Source: CAD feature listing. Evaluate the final solid. Frame: model axes, mm. Give positions to 0.01 mm unless a question says otherwise; leave off trailing zeros. Order: outer loops, then holes, each group sorted by start corner. A loop starts at its lowest first (then second) coordinate and runs counter-clockwise, first axis right, second up. Notation, with made-up numbers: M 17,-9 L 32,-9 A26 cw 32,11 Z; hole C 11,64 d11. An arc over 180 degrees is marked long. One line per question, with ' | ' between items. Start each with the question number.
from build123d import *

# Parameters (mm, degrees)
SKETCH1_R                                       = 335
SKETCH1_R_2                                     = 295
BOSS_EXTRUDE1_DEPTH                             = 8.5
CBORE_FOR_M4_SHCS1_D                            = 4.5
CBORE_FOR_M4_SHCS1_CBORE_D                      = 8
CBORE_FOR_M4_SHCS1_CBORE_DEPTH                  = 4
CSK_FOR_M4_FLAT_HEAD_MACHINE_SCREW1_D           = 4.5
CSK_FOR_M4_FLAT_HEAD_MACHINE_SCREW1_CSINK_D     = 9.4
CSK_FOR_M4_FLAT_HEAD_MACHINE_SCREW1_CSINK_ANGLE = 90


with BuildPart() as part:
    # Sketch1 → Boss-Extrude1 (new body)
    with BuildSketch(Plane(origin=(0, 0, 0), x_dir=(1, 0, 0), z_dir=(0, 1, 0))):
        Circle(SKETCH1_R)
        Circle(SKETCH1_R_2, mode=Mode.SUBTRACT)
    extrude(amount=BOSS_EXTRUDE1_DEPTH)

    # CBORE for M4 SHCS1 (through all)
    with Locations(Plane(origin=(-255.59713911, 32.5, 6.312571873), x_dir=(-0.922302375, 0, -0.386469054), z_dir=(0, 1, 0))):
        with Locations((-208.121459337, -408.561577194), (-34.267123624, -335.712018853), (63.564092484, -174.586473543), (48.003989595, 13.270576883), (-75.004001856, 156.104124188), (-258.475010022, 199.356608036), (-432.329345735, 126.507049694), (-530.160561843, -34.618495616), (-514.600458954, -222.475546041), (-391.592467503, -365.309093346)):
            CounterBoreHole(CBORE_FOR_M4_SHCS1_D / 2, CBORE_FOR_M4_SHCS1_CBORE_D / 2, CBORE_FOR_M4_SHCS1_CBORE_DEPTH)

    # CSK for M4 Flat Head Machine Screw1 (through all)
    with Locations(Plane(origin=(68.292311883, 8.5, -24.828551781), x_dir=(1, 0, 0), z_dir=(0, 1, 0))):
        with Locations((-375.726730436, -130.228164158), (-378.9643189, 70.606787878), (-263.535760038, 234.988683892), (-73.530840061, 300.129226742), (118.475019629, 241.146943105), (239.14210667, 80.571060596), (242.379695134, -120.26389144), (126.951136271, -284.645787454), (-63.053783706, -349.786330304), (-255.059643396, -290.804046667), (-359.846041546, -114.390947461), (-356.807689294, 74.084930603), (-243.566269149, 224.779220342), (-63.376154671, 280.131824986), (114.936154846, 218.999930927), (223.261417779, 64.733843899), (220.223065528, -123.742034166), (106.981645382, -274.436323905), (-73.208469096, -329.788928549), (-251.520778613, -268.65703449)):
            CounterSinkHole(CSK_FOR_M4_FLAT_HEAD_MACHINE_SCREW1_D / 2, CSK_FOR_M4_FLAT_HEAD_MACHINE_SCREW1_CSINK_D / 2, counter_sink_angle=CSK_FOR_M4_FLAT_HEAD_MACHINE_SCREW1_CSINK_ANGLE)


solid = part.part
Item 1: Pin query (flat end, axial travel): pin 1 Ø3.5 at (x, z) = (175.27, 249.61) entering from -Y; pin 2 Ø6 at (x, z) = (186.77, -265.98) entering from +Y; pin 3 Ø2 at (y, z) = (6.5, -105.5) entering from +X; pin 4 Ø1 at (y, z) = (2, -56) entering from -X. Return the tip coordinate at first contact, or that it passes through.
Item 2: Cut plane A-A on z = -152. Return the cut outline in (x, y).
Item 3: Mould query, pull axis X, two halves, no side actions, for faces 1 (the cylindrical face through (-63.95, 4.19, 287.985)), 2 (the cylindrical face through (-265.845, 4.19, 203.842)), 3 (the flat face through (-2, 0, 296)). Classes: pulls with the +X half, pulls with the -X half, needs draft (parallel to the pull), parting line crosses it, or undercut.
Item 4: Cut plane B-B on x = 228. Return the cut outline in (y, z), and give its area (3 significant figures).
Item 5: Line query: line 1 (X direction, y = 5.5, z = 217); line 2 (Z direction, x = 245, y = 0.75); line 3 (Z direction, x = -307, y = 2). Output: solid intervals per line, ascending.
Item 6: Cut plane C-C on y = 3. Count the separate pieces of the cut face and the enclosed holes in it, and give its area (3 significant figures).
Results are:
1) pin 1: passes through | pin 2: stops at y = 6.81 | pin 3: stops at x = 318.28 | pin 4: stops at x = -330.37
2) outline: M -298.53,0 L -252.83,0 L -252.83,8.5 L -298.53,8.5 Z; M 252.83,0 L 298.53,0 L 298.53,8.5 L 252.83,8.5 Z
3) face 1: undercut | face 2: parting line crosses it | face 3: needs draft
4) outline: M 0,-245.44 L 8.5,-245.44 L 8.5,-187.19 L 0,-187.19 Z; M 0,187.19 L 8.5,187.19 L 8.5,245.44 L 0,245.44 Z | area: 990 mm2
5) line 1: x = -255.22 to -199.84, 199.84 to 255.22 | line 2: z = -228.47 to -180.69, -177.86 to -164.32, 164.32 to 177.86, 180.69 to 228.47 | line 3: z = -134.07 to -1.03, 1.03 to 103.19, 107.61 to 134.07
6) separate pieces: 1 | enclosed holes: 31 | area: 78,700 mm2
